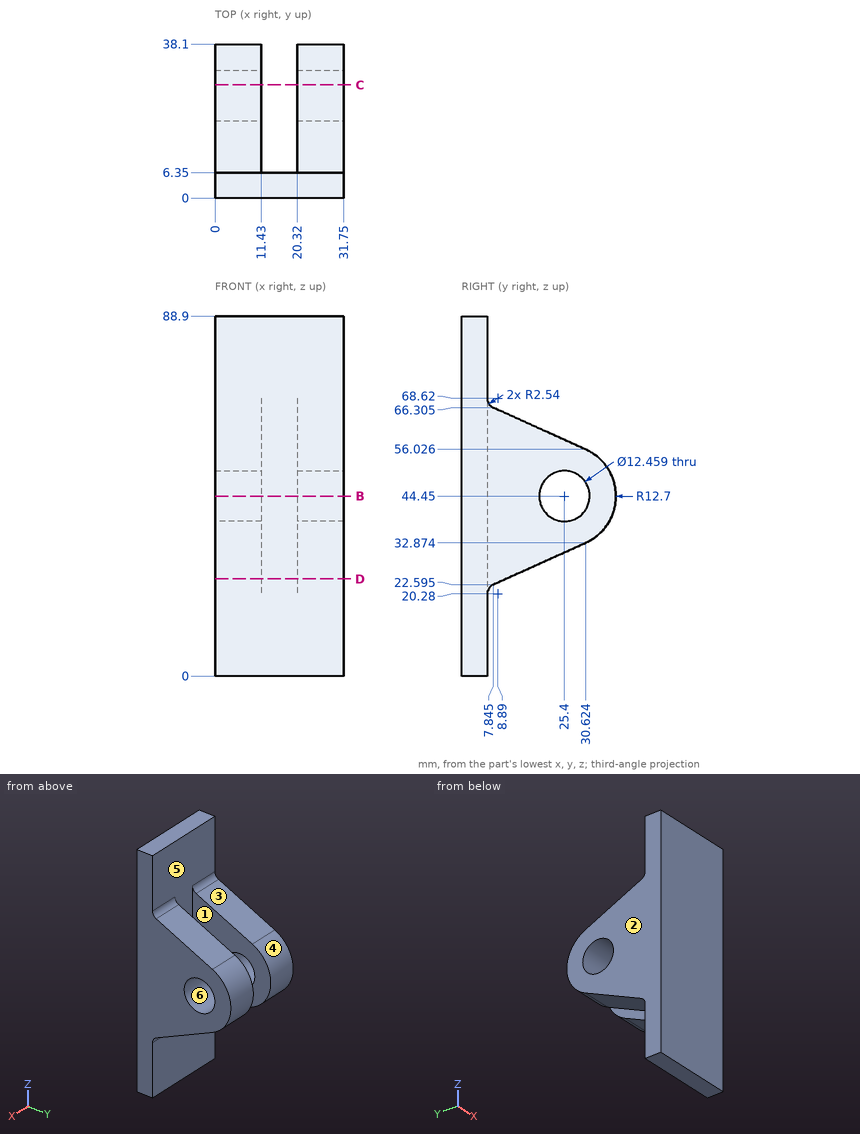
The figure shows three views and two pictorial views of one solid part (mm, origin at its lowest corner). Answer the questions. A direction names the side the tool comes from. Give positions to 0.01 mm unless a question says otherwise; leave off trailing zeros. Write each loop counter-clockwise with the first axis right and the second up, starting at its lowest first coordinate (ties: lowest second). Pieces come first, ordered by that corner, then holes. Notation, with made-up numbers: (58.25, 80.5) - (112.25, 80.5) arc R17 cw to (112.25, 104.5) - close; hole circle Ø2 at (17, 45.25). An arc over 180 degrees is marked (long way). Use one line per item in the form item = value. Start each with the question number.
1) The mould has two halves that part along Z. Classify the marked faces 3, 4, 5 and 6: pulls with the +Z half, pulls with the -Z half, needs draft (parallel to the pull), parting line crosses it, or undercut.
2) Consider line 1 along Y through (x, z) = (4, 44.45); line 2 along X through (y, z) = (34, 43.5); line 3 along Y through (x, z) = (16.5, 73). Determine where each line is inside the solid, lowest interval first. Write a range as from..to.
3) Find section B-B on z = 44.45. Determine the outline of the cut face in (x, y).
4) Find section C-C on y = 28. Determine the outline of the cut face in (x, z).
5) Flat-ended cylindrical pins translate along their axes: pin 1 Ø2 at (x, z) = (14.5, 47.5) entering from +Y; pin 2 Ø16 at (x, z) = (23.5, 31.5) entering from +Y (1 decimal); pin 3 Ø8 at (x, y) = (4, 21.5) entering from -Z. Find the tip coordinate at first contact, or state that the pin passes through.
6) Find section D-D on z = 24. Determine the outline of the cut face in (x, y).
7) A tool of negligible diameter and unlimited length cuts with its end or side. For the marked faces 1 and 2, from which of +Z, -Z, +X, -X, +Y, -Y can it reach the whole face along a straight path? Write none if from no direction.
Geometry results:
q1.face_3 = pulls with the +Z half
q1.face_4 = parting line crosses it
q1.face_5 = needs draft
q1.face_6 = undercut
q2.line_1 = 0..19.17, 31.63..38.1
q2.line_2 = 0..11.43, 20.32..31.75
q2.line_3 = 0..6.35
q3.outline = (0, 0) - (31.75, 0) - (31.75, 19.17) - (20.32, 19.17) - (20.32, 6.35) - (11.43, 6.35) - (11.43, 19.17) - (0, 19.17) - close; (0, 31.63) - (11.43, 31.63) - (11.43, 38.1) - (0, 38.1) - close; (20.32, 31.63) - (31.75, 31.63) - (31.75, 38.1) - (20.32, 38.1) - close
q4.outline = (0, 31.69) - (11.43, 31.69) - (11.43, 38.79) - (0, 38.79) - close; (0, 50.11) - (11.43, 50.11) - (11.43, 57.21) - (0, 57.21) - close; (20.32, 31.69) - (31.75, 31.69) - (31.75, 38.79) - (20.32, 38.79) - close; (20.32, 50.11) - (31.75, 50.11) - (31.75, 57.21) - (20.32, 57.21) - close
q5.pin_1 = 6.35
q5.pin_2 = 37.1
q5.pin_3 = 26.95
q6.outline = (0, 0) - (31.75, 0) - (31.75, 10.96) - (20.32, 10.96) - (20.32, 6.35) - (11.43, 6.35) - (11.43, 10.96) - (0, 10.96) - close
q7.face_1 = +Z, -Z, +Y
q7.face_2 = +Z, -Z, -X, +Y, -Y
